```python
from build123d import *

# Parameters (mm, degrees)
F1_DEPTH = 25.4
F2_R     = 6.35
F3_DEPTH = 25.401
F5_DEPTH = 25.401
F7_DEPTH = 12.701


# Not quite as in the source:
# - a feature names something its author has since deleted; it is built from what else it names


with BuildPart() as f1:
    # F0 (on Front) → F1 (new body)
    with BuildSketch(Plane.XZ):
        Polygon((-46.455263897, 38.1), (-71.855263897, 38.1), (-71.855263897, 0), (-2.005263897, 0), (-2.005263897, 12.7), (-46.455263897, 12.7), align=None)
    extrude(amount=F1_DEPTH)

    # F2 (on face) → F3 (cut, through all)
    with BuildSketch(Plane.XZ.offset(25.4)):
        with Locations((-59.155263897, 25.4)):
            Circle(F2_R)
    extrude(amount=-F3_DEPTH, mode=Mode.SUBTRACT)

    # F4 (on face) → F5 (cut, through all)
    with BuildSketch(Plane.XZ.offset(25.4)):
        with BuildLine():
            ThreePointArc((-71.855263897, 25.4), (-68.135520018, 34.3802561211), (-59.155263897, 38.1))
            Line((-59.155263897, 38.1), (-71.855263897, 38.1))
            Line((-71.855263897, 38.1), (-71.855263897, 25.4))
        make_face()
        with BuildLine():
            ThreePointArc((-59.155263897, 38.1), (-50.1750077759, 34.3802561211), (-46.455263897, 25.4))
            Line((-46.455263897, 25.4), (-46.455263897, 38.1))
            Line((-46.455263897, 38.1), (-59.155263897, 38.1))
        make_face()
    extrude(amount=-F5_DEPTH, mode=Mode.SUBTRACT)

    # F6 (on face) → F7 (cut, through all)
    with BuildSketch(Plane.XY.offset(12.7)):
        with BuildLine():
            ThreePointArc((-13.507871342, -6.3510340362), (-13.6221384518, -6.3500000083), (-13.7364056666, -6.3510223648))
            Line((-13.7364056666, -6.3510223648), (-13.507871342, -6.3510340362))
        make_face()
        with BuildLine():
            Line((-13.507871342, -6.3510340362), (-13.7364056666, -6.3510223648))
            ThreePointArc((-13.7364056666, -6.3510223648), (-19.9722112621, -12.7565139443), (-13.6233824013, -19.0499999334))
            ThreePointArc((-13.6233824013, -19.0499999334), (-9.1326598467, -17.1904531948), (-7.2724627495, -12.7))
            ThreePointArc((-7.2724627495, -12.7), (-9.0920016561, -8.2505705668), (-13.507871342, -6.3510340362))
        make_face()
        with BuildLine():
            ThreePointArc((-33.7549395993, -6.3500000083), (-29.2650211814, -8.2099865975), (-27.405263897, -12.7))
            ThreePointArc((-27.405263897, -12.7), (-29.1979362777, -17.1219073906), (-33.5637725492, -19.0471120255))
            Line((-33.5637725492, -19.0471120255), (-13.6233824013, -19.0499999334))
            ThreePointArc((-13.6233824013, -19.0499999334), (-19.9722112621, -12.7565139443), (-13.7364056666, -6.3510223648))
            Line((-13.7364056666, -6.3510223648), (-33.7549395993, -6.3500000083))
        make_face()
        with BuildLine():
            ThreePointArc((-33.5637725492, -19.0471120255), (-29.1979362777, -17.1219073906), (-27.405263897, -12.7))
            ThreePointArc((-27.405263897, -12.7), (-29.2650211814, -8.2099865975), (-33.7549395993, -6.3500000083))
            ThreePointArc((-33.7549395993, -6.3500000083), (-40.1045443054, -12.7955944315), (-33.5637725492, -19.0471120255))
        make_face()
        with BuildLine():
            ThreePointArc((-13.507871342, 0), (-2.1464755419, -12.7515151154), (-13.6224627495, -25.4))
            Line((-13.6224627495, -25.4), (-2.005263897, -25.4))
            Line((-2.005263897, -25.4), (-2.005263897, 0))
            Line((-2.005263897, 0), (-13.507871342, 0))
        make_face()
    extrude(amount=-F7_DEPTH, mode=Mode.SUBTRACT)


solid = f1.part
```
Can you work these out from the model? Positions are in its coordinate system, mm. A direction names the side the tool comes from. Coordinates: 2 decimals unless noted, no trailing zeros. Loops run counter-clockwise (first coordinate to the right, second up) from the corner with the lowest first, then second, coordinate; pieces in that order, holes last. Notation, with made-up numbers: (-7.75, 10.5) -> (5.25, 10.5) arc R25 ccw to (5.25, 48.5) -> close; hole circle Ø2 at (-21, 20.25). An arc over 180 degrees is marked (long way). Answer as a JSON object with one key per item and string values.
1) Imagine slicing it at A-A (y = -16). Please give me the cut outline in (x, z), then the cut area to 3 significant figures.
Results:
{"outline": "(-71.86, 0) -> (-39.18, 0) -> (-39.18, 12.7) -> (-46.46, 12.7) -> (-46.46, 25.4) arc R12.7 ccw to (-71.86, 25.4) -> close; (-8.2, 0) -> (-2.58, 0) -> (-2.58, 12.7) -> (-8.2, 12.7) -> close; hole circle Ø12.7 at (-59.16, 25.4)", "area": "936 mm^2"}
2) Thinking about a two-plate mould opening in Z: for faces 4 (the face through (-53.29, -12.88, 22.97)), 5 (the face through (-45, -13, 0)), 6 (the face through (-50, 0, 15)), which applies, pulls with the +Z half, pulls with the -Z half, needs draft (parallel to the pull), parting line crosses it, or undercut?
Results:
{"face 4": "undercut", "face 5": "pulls with the -Z half", "face 6": "needs draft"}
3) Imagine slicing it at C-C (z = 23). Please give me the cut outline in (x, y).
Results:
{"outline": "(-71.86, -25.4) -> (-65.03, -25.4) -> (-65.03, 0) -> (-71.86, 0) -> close; (-53.28, -25.4) -> (-46.46, -25.4) -> (-46.46, 0) -> (-53.28, 0) -> close"}
4) For faces 1 (the face through (-40.105, -12.655, 6.439)), 2 (the face through (-24, -21, 12.7)), 3 (the face through (-71.855, -13, 13)), which set-ups out of +Z, -Z, +X, -X, +Y, -Y let a thin tool reach every point of the face, with its end or its side?
Results:
{"face 1": "+Z, -Z", "face 2": "+Z, +X, +Y, -Y", "face 3": "+Z, -Z, -X, +Y, -Y"}
5) Imagine slicing it at D-D (z = 5). Please give me the cut outline in (x, y), then the cut area to 3 significant figures.
Results:
{"outline": "(-71.86, -25.4) -> (-13.62, -25.4) arc R12.77 ccw to (-13.51, 0) -> (-71.86, 0) -> close; hole (-33.75, -6.35) arc R6.35 ccw (long way) to (-33.56, -19.05) -> (-13.62, -19.05) arc R6.35 ccw (long way) to (-13.74, -6.35) -> close", "area": "1,320 mm^2"}
6) Imagine slicing it at B-B (x = -37). Please give me the cut outline in (y, z).
Results:
{"outline": "(-25.4, 0) -> (-18.16, 0) -> (-18.16, 12.7) -> (-25.4, 12.7) -> close; (-7.24, 0) -> (0, 0) -> (0, 12.7) -> (-7.24, 12.7) -> close"}
7) For P1, Ø2, axis at x = -60.5, z = 29, coming from the +Y side; P2, Ø14, axis at y = -9.5, z = 17.5, coming from the +X side; P3, Ø2, axis at x = -64, y = -22.5, coming from the +Z side, each with a flat end and sliding along its axis, tell me the tip position at first contact or that it passes through.
Results:
{"P1": "passes through", "P2": "stops at x = -2.15", "P3": "stops at z = 37.5"}
8) If I drill on line 1 (X direction, y = -12.75, z = 3); line 2 (Z direction, x = -45, y = -9); line 3 (X direction, y = -7, z = 13), over which ranges is the centre line in solid material (lowest first)?
Results:
{"line 1": "x = -71.86 to -40.11, -7.27 to -2.15", "line 2": "z = 0 to 12.7", "line 3": "x = -71.86 to -46.46"}
